Design review of the part shown in the three views and the two pictorial views. Dimensions are in mm from the part's minimum x, y and z. Round coordinates to 2 decimals unless told otherwise and drop trailing zeros. Loops run counter-clockwise (first coordinate to the right, second up) from the corner with the lowest first, then second, coordinate; pieces in that order, holes last. Notation, with made-up numbers: M 32,-7.5 L 76,-7.5 A20 cw 76,21.5 Z; hole C -2,-33 d5. An arc over 180 degrees is marked long. One line per question, with ' | ' between items. Start each with the question number.
1) We need section D-D (x = 15.75). Give the boundary of the cut face in (y, z).
2) For pin 1 Ø5 at (y, z) = (14.5, 10.5) entering from -X; pin 2 Ø6 at (y, z) = (10.5, 8.5) entering from +X; pin 3 Ø5 at (x, z) = (12, 7) entering from -Y, all flat-tipped, find the tip position at first contact; note any pin that passes through.
3) For probe 1 along Y at (x, z) = (9, 9.25); probe 2 along X at (y, z) = (5.5, 4); probe 3 along X at (y, z) = (7.25, 7.25), list the stretches that pass through material, from the lowest coordinate up. Write a range as from..to.
4) Mouldability with a two-part tool opening along Y and no side actions: class the marked faces 1, 2 and 3 as pulls with the +Y half, pulls with the -Y half, needs draft (parallel to the pull), parting line crosses it, or undercut.
5) We need section C-C (z = 1.75). Give the boundary of the cut face in (x, y), and give its area (3 significant figures).
6) We need section A-A (x = 9). Give the boundary of the cut face in (y, z), and give its area (3 significant figures).
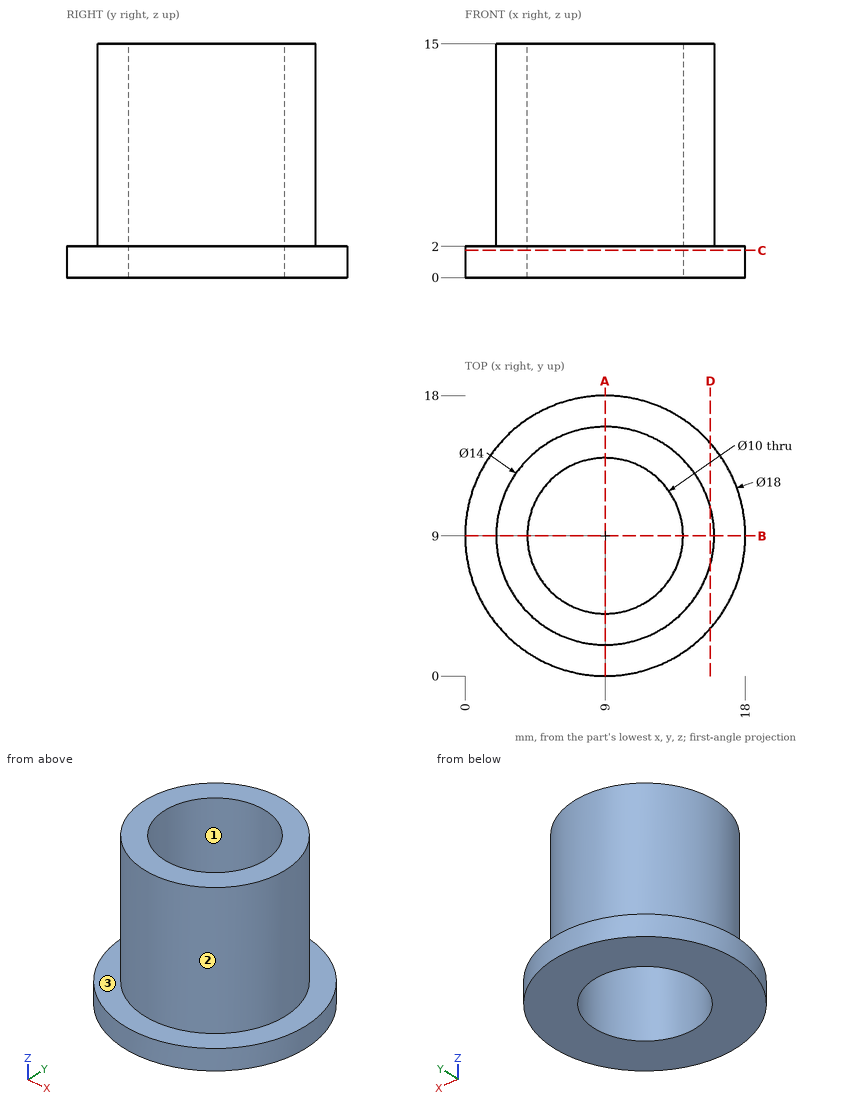
Answers below:
1) outline: M 3.05,0 L 14.95,0 L 14.95,2 L 10.85,2 L 10.85,15 L 7.15,15 L 7.15,2 L 3.05,2 Z
2) pin 1: x = 2.68 | pin 2: x = 16 | pin 3: y = 2.02
3) probe 1: 2..4, 14..16 | probe 2: 2.94..5.43, 12.57..15.06 | probe 3: 2.22..4.32, 13.68..15.78
4) face 1: undercut | face 2: parting line crosses it | face 3: needs draft
5) outline: C 9,9 d18; hole C 9,9 d10 | area: 176 mm^2
6) outline: M 0,0 L 4,0 L 4,15 L 2,15 L 2,2 L 0,2 Z; M 14,0 L 18,0 L 18,2 L 16,2 L 16,15 L 14,15 Z | area: 68.0 mm^2
